Here's how the part is built. I have some questions about the finished solid (model axes, mm). A direction names the side the tool comes from. Give positions to 0.01 mm unless a question says otherwise; leave off trailing zeros. Loops run counter-clockwise (first coordinate to the right, second up) from the corner with the lowest first, then second, coordinate; pieces in that order, holes last. Notation, with made-up numbers: (-31, -4.5) - (2, -4.5) arc R20 ccw to (2, 3.5) - close; hole circle Ø6 at (88.25, 28.5). An arc over 180 degrees is marked (long way). Put each result on its own line as item: value. Start each with the question number.
from build123d import *

# Parameters (mm, degrees)
SKETCH1_W           = 50.8
SKETCH1_H           = 45.72
SKETCH1_W_2         = 32.004
SKETCH1_H_2         = 12.192
BOSS_EXTRUDE1_DEPTH = 12.7
BOSS_EXTRUDE2_START = -22.86
SKETCH2_R           = 1.671921998
BOSS_EXTRUDE2_DEPTH = 6.35
BOSS_EXTRUDE3_START = -16.51
SKETCH4_R           = 0.6
BOSS_EXTRUDE3_DEPTH = 3.556
BOSS_EXTRUDE4_DEPTH = 3.175
BOSS_EXTRUDE5_START = 3.175
SKETCH6_W           = 4.454
SKETCH6_H           = 12.192
BOSS_EXTRUDE5_DEPTH = 3.556
BOSS_EXTRUDE6_START = 22.86
BOSS_EXTRUDE6_DEPTH = 6.35
BOSS_EXTRUDE7_START = 22.86
SKETCH8_R           = 3.745494863
BOSS_EXTRUDE7_DEPTH = 4.826


with BuildPart() as part:
    # Sketch1 → Boss-Extrude1 (new body)
    with BuildSketch(Plane(origin=(0, 0, 0), x_dir=(1, 0, 0), z_dir=(0, 1, 0))):
        Rectangle(SKETCH1_W, SKETCH1_H)
        Rectangle(SKETCH1_W_2, SKETCH1_H_2, mode=Mode.SUBTRACT)
    extrude(amount=BOSS_EXTRUDE1_DEPTH)

    # Sketch2 → Boss-Extrude2 (add)
    # profile 1 of 2: a face of its own
    with BuildSketch(Plane.XY.offset(BOSS_EXTRUDE2_START)):
        with BuildLine():
            Line((-6.020374567, 38.1), (-6.020374567, 25.4))
            Line((-6.020374567, 25.4), (-18.720374567, 25.4))
            Line((-18.720374567, 25.4), (-25.4, 19.05))
            Line((-25.4, 19.05), (-25.4, 12.7))
            Line((-25.4, 12.7), (-19.05, 12.7))
            Line((-19.05, 12.7), (-19.05, 16.325160807))
            Line((-19.05, 16.325160807), (-16.18371572, 19.05))
            Line((-16.18371572, 19.05), (-6.020374567, 19.05))
            Line((-6.020374567, 19.05), (-6.020374567, 12.7))
            Line((-6.020374567, 12.7), (6.679625433, 12.7))
            Line((6.679625433, 12.7), (6.679625433, 19.05))
            Line((6.679625433, 19.05), (16.842966586, 19.05))
            Line((16.842966586, 19.05), (19.05, 16.951879032))
            Line((19.05, 16.951879032), (19.05, 12.7))
            Line((19.05, 12.7), (25.4, 12.7))
            Line((25.4, 12.7), (25.4, 19.676718225))
            Line((25.4, 19.676718225), (19.379625433, 25.4))
            Line((19.379625433, 25.4), (6.679625433, 25.4))
            Line((6.679625433, 25.4), (6.679625433, 38.1))
            ThreePointArc((6.679625433, 38.1), (0.329625433, 44.45), (-6.020374567, 38.1))
        make_face()
        with BuildLine():
            Line((-2.296540764, 35.862646406), (-1.515493151, 23.920283336))
            ThreePointArc((-1.515493151, 23.920283336), (0.501683423, 22.050922268), (2.478319103, 23.963099958))
            Line((2.478319103, 23.963099958), (3.003154686, 35.919463063))
            ThreePointArc((3.003154686, 35.919463063), (0.292641005, 41.549801755), (-2.296540764, 35.862646406))
        make_face(mode=Mode.SUBTRACT)
    # profile 2 of 2: a face of its own
    with BuildSketch(Plane.XY.offset(BOSS_EXTRUDE2_START)):
        with Locations((0.329625433, 38.1)):
            Circle(SKETCH2_R)
    extrude(amount=BOSS_EXTRUDE2_DEPTH)


with BuildPart() as boss_extrude2_kept_piece:
    # of the separate pieces the step leaves, the one the design keeps (boss_extrude2_pieces_kept)
    add(part.part.solids().sort_by_distance((-25.4, 0, 22.86))[0])

    # Sketch4 → Boss-Extrude3 (add)
    with BuildSketch(Plane.XY.offset(BOSS_EXTRUDE3_START)):
        with BuildLine():
            ThreePointArc((-1.515493151, 23.920283336), (0.501683423, 22.050922268), (2.478319103, 23.963099958))
            Line((2.478319103, 23.963099958), (3.003154686, 35.919463063))
            ThreePointArc((3.003154686, 35.919463063), (0.366609861, 34.650198245), (-2.296540764, 35.862646406))
            Line((-2.296540764, 35.862646406), (-1.515493151, 23.920283336))
        make_face()
        with Locations((0.484531225, 23.650830329)):
            Circle(SKETCH4_R, mode=Mode.SUBTRACT)
        with Locations((0.441650729, 27.65060048)):
            Circle(SKETCH4_R, mode=Mode.SUBTRACT)
        with Locations((0.398770233, 31.650370631)):
            Circle(SKETCH4_R, mode=Mode.SUBTRACT)
    extrude(amount=-BOSS_EXTRUDE3_DEPTH)

    # Sketch5 → Boss-Extrude4 (add)
    with BuildSketch(Plane(origin=(0, 0, 0), x_dir=(1, 0, 0), z_dir=(0, 1, 0))):
        with BuildLine():
            Line((16.002, 6.354), (5.198, 6.354))
            ThreePointArc((5.198, 6.354), (11.548, 0.004), (5.198, -6.346))
            Line((5.198, -6.346), (16.002, -6.346))
            Line((16.002, -6.346), (16.002, 6.354))
        make_face()
        with BuildLine():
            ThreePointArc((-0.302167411, 3.177430077), (2.022215136, 5.502808098), (5.198, 6.354))
            Line((5.198, 6.354), (-16.002, 6.354))
            Line((-16.002, 6.354), (-16.002, -6.346))
            Line((-16.002, -6.346), (5.198, -6.346))
            ThreePointArc((5.198, -6.346), (2.022215136, -5.494808098), (-0.302167411, -3.169430077))
            ThreePointArc((-0.302167411, -3.169430077), (-3.577, 0.004), (-0.302167411, 3.177430077))
        make_face()
    extrude(amount=BOSS_EXTRUDE4_DEPTH)

    # Sketch6 → Boss-Extrude5 (add)
    with BuildSketch(Plane(origin=(0, 0, 0), x_dir=(1, 0, 0), z_dir=(0, 1, 0)).offset(BOSS_EXTRUDE5_START)):
        with Locations((-13.775, 0)):
            Rectangle(SKETCH6_W, SKETCH6_H)
        with Locations((13.775, 0)):
            Rectangle(SKETCH6_W, SKETCH6_H)
    extrude(amount=BOSS_EXTRUDE5_DEPTH)



with BuildPart() as body_2:
    # Sketch7 → Boss-Extrude6 (new body)
    with BuildSketch(Plane.XY.offset(BOSS_EXTRUDE6_START)):
        with BuildLine():
            Line((-6.020374567, 12.7), (6.679625433, 12.7))
            Line((6.679625433, 12.7), (6.679625433, 19.05))
            Line((6.679625433, 19.05), (16.842966586, 19.05))
            Line((16.842966586, 19.05), (19.05, 16.951879032))
            Line((19.05, 16.951879032), (19.05, 12.7))
            Line((19.05, 12.7), (25.4, 12.7))
            Line((25.4, 12.7), (25.4, 19.676718225))
            Line((25.4, 19.676718225), (19.379625433, 25.4))
            Line((19.379625433, 25.4), (4.075120296, 25.475))
            Line((4.075120296, 25.475), (4.075120296, 38.1))
            ThreePointArc((4.075120296, 38.1), (0.329625433, 41.845494863), (-3.41586943, 38.1))
            Line((-3.41586943, 38.1), (-3.41586943, 25.475))
            Line((-3.41586943, 25.475), (-18.720374567, 25.4))
            Line((-18.720374567, 25.4), (-25.4, 19.05))
            Line((-25.4, 19.05), (-25.4, 12.7))
            Line((-25.4, 12.7), (-19.05, 12.7))
            Line((-19.05, 12.7), (-19.05, 16.325160807))
            Line((-19.05, 16.325160807), (-16.18371572, 19.05))
            Line((-16.18371572, 19.05), (-6.020374567, 19.05))
            Line((-6.020374567, 19.05), (-6.020374567, 12.7))
        make_face()
    extrude(amount=-BOSS_EXTRUDE6_DEPTH)


with BuildPart() as boss_extrude2_kept_piece_1:
    add(boss_extrude2_kept_piece.part)

    add(body_2.part)  # Boss-Extrude7 merges body 2
    # Sketch8 → Boss-Extrude7 (add)
    with BuildSketch(Plane.XY.offset(BOSS_EXTRUDE7_START)):
        with Locations(Location((0.329625433, 38.1, 0), (0, 0, 180))):
            Circle(SKETCH8_R)
    extrude(amount=BOSS_EXTRUDE7_DEPTH)


solid = boss_extrude2_kept_piece_1.part
1) I need wall thicknesses on line 1 (Z direction, x = 1, y = 10); line 2 (Z direction, x = -12.5, y = 19.5); line 3 (X direction, y = 38.1, z = -18.25). Which ranges of each line are inside material? Lowest first, please.
2) Suppose I cut it at B-B on y = 33. Please give me the cut outline in (x, z) (3 decimals), plus the area to 3 significant figures.
3) Which directions (+Z, -Z, +X, -X, +Y, -Y) give clear straight access to the entire face, cutting with the end or side of a thin tool? Please do faces 4 (the flat face through (12, 19.05, 20)), 5 (the cylindrical face through (1.24, 1.57, -4.97)), 6 (the flat face through (-11.548, 5, 0)).
4) Suppose I cut it at A-A on y = 10. Please give me the cut outline in (x, z).
5) Suppose I cut it at D-D on x = 10.5. Please give me the cut outline in (y, z) (3 decimals).
6) Thinking about a two-plate mould opening in Y: for faces 1 (the flat face through (-12, 25.4, -20)), 2 (the flat face through (-25.4, 8, 0)), 3 (the flat face through (12, 19.05, -20)), which applies, pulls with the +Y half, pulls with the -Y half, needs draft (parallel to the pull), parting line crosses it, or undercut?
7) Suppose I cut it at C-C on z = 17.5. Give the number of separate pieces and of enclosed holes in the cut face, plus the area to 3 significant figures.
8) I'm going to push flat-ended pins straight in: P1, Ø6, axis at x = -18.5, y = 15, coming from the +Z side; P2, Ø7, axis at x = 12.5, z = -20.5, coming from the +Y side; P3, Ø8, axis at x = -6.5, z = 6.5, coming from the +Y side. Where does each tip first touch, or does it pass through?
Ans:
1. line 1: z = -22.86 to -6.1, 6.1 to 22.86
1. line 2: z = -22.86 to -16.51, 16.51 to 22.86
1. line 3: x = -6.02 to -3.12, 3.78 to 6.68
2. outline: (-6.02, -22.86) - (-2.109, -22.86) - (-2.109, -20.066) - (2.875, -20.066) - (2.875, -22.86) - (6.68, -22.86) - (6.68, -16.51) - (-6.02, -16.51) - close; (-3.416, 16.51) - (4.075, 16.51) - (4.075, 22.86) - (-3.416, 22.86) - close
2. area: 114 mm²
3. face 4: +Z, -Z
3. face 5: +Y, -Y
3. face 6: +Y
4. outline: (-25.4, -22.86) - (25.4, -22.86) - (25.4, 22.86) - (-25.4, 22.86) - close; hole (-16, -6.1) - (16, -6.1) - (16, 6.1) - (-16, 6.1) - close
5. outline: (0, -22.86) - (12.7, -22.86) - (12.7, -6.096) - (3.175, -6.096) - (3.175, -3.498) - (0, -3.498) - close; (0, 3.49) - (3.175, 3.49) - (3.175, 6.096) - (12.7, 6.096) - (12.7, 22.86) - (0, 22.86) - close; (19.05, -22.86) - (25.4, -22.86) - (25.4, -16.51) - (19.05, -16.51) - close; (19.05, 16.51) - (25.444, 16.51) - (25.444, 22.86) - (19.05, 22.86) - close
6. face 1: pulls with the +Y half
6. face 2: needs draft
6. face 3: undercut
7. separate pieces: 1
7. enclosed holes: 2
7. area: 1,220 mm²
8. P1: stops at z = 22.86
8. P2: stops at y = 25.4
8. P3: stops at y = 12.7
